Work out the finished part from the listing and answer in its coordinate system (mm). A direction names the side the tool comes from. Round coordinates to 2 decimals unless told otherwise and drop trailing zeros. Order: outer loops, then holes, each group sorted by start corner. A loop starts at its lowest first (then second) coordinate and runs counter-clockwise, first axis right, second up. Notation, with made-up numbers: (-26.5, -9.5) - (5.5, -9.5) arc R25 cw to (5.5, 20.5) - close; hole circle Ø7 at (10.25, 37.25). An arc over 180 degrees is marked (long way). Put each result on its own line as item: value.
```python
from build123d import *

# Parameters (mm, degrees)
BOSS_EXTRU_1_DEPTH = 3


with BuildPart() as part:
    # Esquisse1 → Boss.-Extru.1 (new body)
    with BuildSketch(Plane(origin=(0, 0, 0), x_dir=(1, 0, 0), z_dir=(0, 1, 0))):
        Polygon((-12.05, 36.5), (0, 36.5), (0, 38), (-17.05, 38), (-17.05, 0), (0, 0), (0, 24), (-12.05, 24), align=None)
        with BuildLine():
            ThreePointArc((-15.05, 29.25), (-16.05, 30.25), (-15.05, 31.25))
            Line((-15.05, 31.25), (-14.05, 31.25))
            ThreePointArc((-14.05, 31.25), (-13.05, 30.25), (-14.05, 29.25))
            Line((-14.05, 29.25), (-15.05, 29.25))
        make_face(mode=Mode.SUBTRACT)
    boss_extru_1 = extrude(amount=BOSS_EXTRU_1_DEPTH)

    # Symétrie1: Boss.-Extru.1 across plane
    add(boss_extru_1.mirror(Plane(origin=(0, 3, 0), x_dir=(0, 0, 1), z_dir=(-1, 0, 0))))


solid = part.part
```
1) A cutting plane is placed at C-C on y = 2.55. Write down the section's boundary in (x, z), then the cut area to 3 significant figures.
Findings below:
outline: (-17.05, -38) - (17.05, -38) - (17.05, 0) - (-17.05, 0) - close; hole (-15.05, -31.25) - (-14.05, -31.25) arc R1 ccw to (-14.05, -29.25) - (-15.05, -29.25) arc R1 ccw to start; hole (-12.05, -36.5) - (12.05, -36.5) - (12.05, -24) - (-12.05, -24) - close; hole (14.05, -31.25) - (15.05, -31.25) arc R1 ccw to (15.05, -29.25) - (14.05, -29.25) arc R1 ccw to start
area: 984 mm2
2) For faces 1 (the flat face through (-17.05, 1, -19)), 2 (the cylindrical face through (13.05, 1.48, -30.27)), determine the directions among +Z, -Z, +X, -X, +Y, -Y from which every point of the face is accessible in a straight line to the end or side of a thin tool.
Findings below:
face 1: +Z, -Z, -X, +Y, -Y
face 2: +Y, -Y
3) A cutting plane is placed at A-A on z = -35. Write down the section's boundary in (x, y).
Findings below:
outline: (-17.05, 0) - (-12.05, 0) - (-12.05, 3) - (-17.05, 3) - close; (12.05, 0) - (17.05, 0) - (17.05, 3) - (12.05, 3) - close
4) For a pull along Z with two mould halves and no side action, classify faces 3 (the flat face through (0, 1, -38)), 4 (the flat face through (0, 0, -15)), 5 (the flat face through (0, 1, 0)), 6 (the cylindrical face through (16.05, 1.48, -30.23)) as pulls with the +Z half, pulls with the -Z half, needs draft (parallel to the pull), parting line crosses it, or undercut.
Findings below:
face 3: pulls with the -Z half
face 4: needs draft
face 5: pulls with the +Z half
face 6: undercut
5) Straight lines are drawn through the part: L1, parallel to Z at x = -2, y = 1.35; L2, parallel to Z at x = 14, y = 2.1; L3, parallel to X at y = 0.45, z = -34. For each, find the intervals that lie inside material, in ascending order. Write a range as from..to.
Findings below:
L1: z = -38..-36.5, -24..0
L2: z = -38..-31.25, -29.25..0
L3: x = -17.05..-12.05, 12.05..17.05
6) A cutting plane is placed at B-B on x = -13.5. Write down the section's boundary in (y, z), then the cut area to 3 significant figures.
Findings below:
outline: (0, -38) - (3, -38) - (3, -31.09) - (0, -31.09) - close; (0, -29.41) - (3, -29.41) - (3, 0) - (0, 0) - close
area: 109 mm2
7) Given pin 1 Ø0.5 at (x, y) = (14.5, 2) entering from +Z, flat-ended and moving along its own axis, determine where the tip first touches the part or whether it passes through.
Findings below:
pin 1: stops at z = 0
